from build123d import *

# Parameters (mm, degrees)
BOSS_EXTRUDE1_DEPTH = 26
SKETCH2_R           = 15
SKETCH2_R_2         = 7
BOSS_EXTRUDE2_DEPTH = 30
CUT_EXTRUDE1_REACH  = 75.362
SKETCH3_R           = 7


with BuildPart() as part:
    # Sketch1 → Boss-Extrude1 (new, symmetric)
    with BuildSketch(Plane.XY):
        Polygon((-25, 0), (-9, 0), (-9, 7), (-9, 48), (9, 48), (9, 7), (9, 0), (25, 0), (25, 7), (16, 7), (16, 48), (16, 55), (-16, 55), (-16, 48), (-16, 7), (-25, 7), align=None)
    extrude(amount=BOSS_EXTRUDE1_DEPTH, both=True)

    # Sketch2 → Boss-Extrude2 (add)
    with BuildSketch(Plane(origin=(16, 0, 0), x_dir=(0, 0, -1), z_dir=(1, 0, 0))):
        with Locations(Location((0, 31, 0), (0, 0, 270))):
            Circle(SKETCH2_R)
        with Locations(Location((0, 31, 0), (0, 0, 90))):
            Circle(SKETCH2_R_2, mode=Mode.SUBTRACT)
    extrude(amount=BOSS_EXTRUDE2_DEPTH)

    # Sketch3 → Cut-Extrude1 (cut, up to next)
    with BuildSketch(Plane(origin=(16, 0, 0), x_dir=(0, 0, -1), z_dir=(1, 0, 0)), mode=Mode.PRIVATE) as cut_extrude1_sk1:
        with Locations((0, 31)):
            Circle(SKETCH3_R)
    cut_extrude1_tool1 = extrude(cut_extrude1_sk1.sketch, amount=-CUT_EXTRUDE1_REACH, mode=Mode.PRIVATE) & part.part
    add(cut_extrude1_tool1.solids().sort_by_distance((16, 31, 0))[0], mode=Mode.SUBTRACT)


solid = part.part
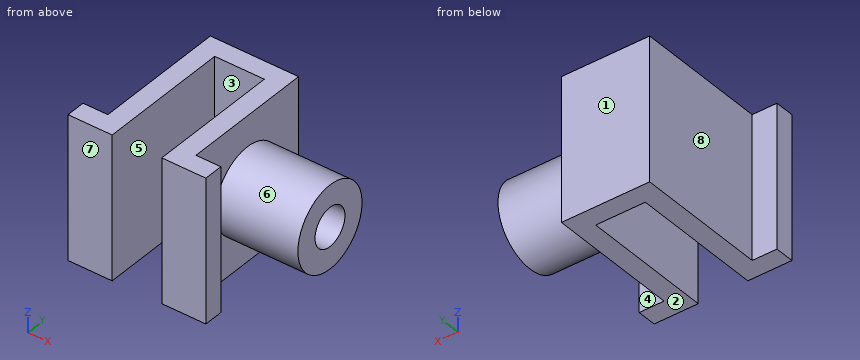
CAD build for the part. Positions are in the model's coordinates, mm. Face numbers are marked on the shaded views. A direction names the side the tool comes from. Give positions to 0.01 mm unless a question says otherwise; leave off trailing zeros. Loops run counter-clockwise (first coordinate to the right, second up) from the corner with the lowest first, then second, coordinate; pieces in that order, holes last. Notation, with made-up numbers: M 31.5,-9.5 L 46.5,-9.5 A28 cw 46.5,25.5 Z; hole C 69.5,-27.5 d1. An arc over 180 degrees is marked long. Answer in a Markdown table with one row per item. Add a question column.
Item 1: Band-saw the part on B-B on x = 18. Give the cut face in (y, z).
Item 2: Mould opens along Y. For the marked faces 1, 2, 3 and 4 say: +Y half, -Y half, draft (parallel to the pull), parting line (faces both ways), or undercut.
Item 3: Drop flat-ended pins along their axis: P1, Ø6, axis at x = 31.5, z = -13.5, coming from the -Y side; P2, Ø8, axis at x = 23, y = 43, coming from the +Z side; P3, Ø24, axis at y = 27, z = 8, coming from the -X side. Give the stop position or say it passes through.
Item 4: Band-saw the part on A-A on y = 31. Give the cut face in (x, z).
Item 5: Probe probe 1 along X at (y, z) = (23, -11); probe 2 along X at (y, z) = (18.5, 17.5); probe 3 along Z at (x, y) = (36, 31). List the from-to ranges inside material, lowest first.
Item 6: Tool access for the marked faces 5, 6, 7 and 8: list every direction of +Z, -Z, +X, -X, +Y, -Y with a clear straight run to the whole face (end or side of a thin tool).
Item 7: Band-saw the part on D-D on y = 22. Give the cut face in (x, z).
Item 8: Band-saw the part on C-C on z = 0. Give the cut face in (x, y).
Reply:
| question | item | result |
|---|---|---|
| 1 | outline | M 0,-26 L 7,-26 L 7,26 L 0,26 Z; C 31,0 d30; hole C 31,0 d14 |
| 2 | face 1 | +Y half |
| 2 | face 2 | draft |
| 2 | face 3 | -Y half |
| 2 | face 4 | undercut |
| 3 | P1 | stops at y = 20.29 |
| 3 | P2 | stops at z = 12.69 |
| 3 | P3 | stops at x = -16 |
| 4 | outline | M -16,-26 L -9,-26 L -9,26 L -16,26 Z; M 9,-26 L 16,-26 L 16,-15 L 46,-15 L 46,-7 L 9,-7 Z; M 9,7 L 46,7 L 46,15 L 16,15 L 16,26 L 9,26 Z |
| 5 | probe 1 | x = -16 to -9, 9 to 46 |
| 5 | probe 2 | x = -16 to -9, 9 to 16 |
| 5 | probe 3 | z = -15 to -7, 7 to 15 |
| 6 | face 5 | +Z, -Z, -Y |
| 6 | face 6 | +X |
| 6 | face 7 | +Z, -Z, +X, -X, -Y |
| 6 | face 8 | +Z, -Z, -X, +Y |
| 7 | outline | M -16,-26 L -9,-26 L -9,26 L -16,26 Z; M 9,-26 L 16,-26 L 16,-12 L 46,-12 L 46,12 L 16,12 L 16,26 L 9,26 Z |
| 8 | outline | M -25,0 L -9,0 L -9,48 L 9,48 L 9,38 L 46,38 L 46,46 L 16,46 L 16,55 L -16,55 L -16,7 L -25,7 Z; M 9,0 L 25,0 L 25,7 L 16,7 L 16,16 L 46,16 L 46,24 L 9,24 Z |
